Here's how the part is built. I have some questions about the finished solid (model axes, mm). A direction names the side the tool comes from. Round coordinates to 2 decimals unless told otherwise and drop trailing zeros. Write each loop counter-clockwise with the first axis right and the second up, starting at its lowest first coordinate (ties: lowest second). Pieces come first, ordered by that corner, then holes. Notation, with made-up numbers: (32.25, 54) -> (76.25, 54) arc R19 cw to (76.25, 74) -> close; hole circle Ø3 at (-36, 44). An arc over 180 degrees is marked (long way). Answer as CSV lines item,"result".
Solid Edge part; units mm, degrees
sketch "Sketch1" plane through (0, 0, 0) normal (0, 0, 1) x (1, 0, 0)
  line L0 (-7.7, -5.4) -> (7.7, -5.4)
  line L1 (7.7, -5.4) -> (7.7, -2.8)
  line L2 (7.7, -2.8) -> (9.7, -2.8)
  arc A0 (9.7, 2.8) -> (9.7, -2.8) centre (9.7, 0) cw
  line L3 (7.7, 2.8) -> (9.7, 2.8)
  line L4 (7.7, 5.4) -> (7.7, 2.8)
  line L5 (7.7, 5.4) -> (-7.7, 5.4)
  line L6 (-7.7, 5.4) -> (-7.7, 2.8)
  line L7 (-7.7, 2.8) -> (-9.7, 2.8)
  arc A1 (-9.7, 2.8) -> (-9.7, -2.8) centre (-9.7, 0) ccw
  line L8 (-7.7, -2.8) -> (-9.7, -2.8)
  line L9 (-7.7, -5.4) -> (-7.7, -2.8)
  dimension "D1" = 7.7
extrude "Protrusion1" add sketch "Sketch1" along normal blind 1.6
sketch "Sketch2" plane through (0, 0, 1.6) normal (0, 0, 1) x (1, 0, 0)
  circle A0 centre (9.65, 0) radius 1.45
  circle A1 centre (-9.65, 0) radius 1.45
extrude "Cutout1" cut sketch "Sketch2" against normal through all
sketch "Sketch3" plane through (0, 0, 1.6) normal (0, 0, 1) x (1, 0, 0)
  circle A0 centre (-6.25, -4.4) radius 0.5
  circle A1 centre (-3.75, -4.4) radius 0.5
  circle A2 centre (-1.25, -4.4) radius 0.5
  circle A3 centre (1.25, -4.4) radius 0.5
  circle A4 centre (3.75, -4.4) radius 0.5
  circle A5 centre (6.25, -4.4) radius 0.5
extrude "Cutout2" cut sketch "Sketch3" against normal through all
sketch "Sketch4" plane through (0, 0, 1.6) normal (0, 0, 1) x (1, 0, 0)
  line L0 (-2.5, 1.1) -> (2.5, 1.1)
  line L1 (2.5, 1.1) -> (2.5, 4.1)
  line L2 (2.5, 4.1) -> (-2.5, 4.1)
  line L3 (-2.5, 4.1) -> (-2.5, 1.1)
  dimension "D1" = 2.5
  dimension "D2" = 2.5
extrude "Extrusionsausprägung_2" add sketch "Sketch4" along normal blind 1.5
sketch "Sketch5" plane through (0, 0, 0) normal (0, 0, -1) x (-1, 0, 0)
  line L0 (-7.7, 5.4) -> (7.7, 5.4)
  line L1 (7.7, 5.4) -> (7.7, -2.9)
  line L2 (7.7, -2.9) -> (-7.7, -2.9)
  line L3 (-7.7, -2.9) -> (-7.7, 5.4)
extrude "Extrusionsausprägung_3" add sketch "Sketch5" along normal blind 1.5
Item 1: Suppose I cut it at B-B, the plane z = 0.65. State how many separate pieces and enclosed holes the cut face has, then the cut area to 3 significant figures.
Results found:
separate pieces,"1"
enclosed holes,"8"
area,"195 mm²"
Item 2: Suppose I cut it at A-A, the plane x = -6.25. List the corners of the cut face in (y, z) for me.
Results found:
outline,"(-5.4, 0) -> (-4.9, 0) -> (-4.9, 1.6) -> (-5.4, 1.6) -> close; (-3.9, 0) -> (-2.9, 0) -> (-2.9, -1.5) -> (5.4, -1.5) -> (5.4, 1.6) -> (-3.9, 1.6) -> close"
Item 3: Will these pins go through, and if not, where does the flat tip stop? pin 1 (4 mm diameter, centred on x = -9.65, y = 0, fed in from +Z); pin 2 (1.6 mm diameter, centred on y = 2, z = 2.5, fed in from +X); pin 3 (0.8 mm diameter, centred on x = -8.5, z = 0.5, fed in from -Y); pin 4 (1.7 mm diameter, centred on x = 9.65, y = 0, fed in from -Z).
Results found:
pin 1,"stops at z = 1.6"
pin 2,"stops at x = 2.5"
pin 3,"stops at y = -2.8"
pin 4,"passes through"
Item 4: For faces 4 (the flat face through (9, 2.8, 1)), 5 (the flat face through (-11, 1, 0)), 6 (the flat face through (2.5, 3, 2)), 7 (the flat face through (0, 1.1, 2)), 8 (the flat face through (0, -2.9, -1)), which set-ups out of +Z, -Z, +X, -X, +Y, -Y let a thin tool reach every point of the face, with its end or its side?
Results found:
face 4,"+Z, -Z, +X, +Y"
face 5,"-Z, -X, +Y, -Y"
face 6,"+Z, +X, +Y, -Y"
face 7,"+Z, +X, -X, -Y"
face 8,"-Z, +X, -X, -Y"
Item 5: Suppose I cut it at D-D, the plane x = -2. List the corners of the cut face in (y, z) for me.
Results found:
outline,"(-5.4, 0) -> (-2.9, 0) -> (-2.9, -1.5) -> (5.4, -1.5) -> (5.4, 1.6) -> (4.1, 1.6) -> (4.1, 3.1) -> (1.1, 3.1) -> (1.1, 1.6) -> (-5.4, 1.6) -> close"
Item 6: I need wall thicknesses on L1, parallel to Y at x = -1.25, z = 0.9; L2, parallel to Y at x = -9.65, z = 0.4; L3, parallel to Z at x = 2.5, y = 1. Which ranges of each line are inside material? Lowest first, please.
Results found:
L1,"y = -5.4 to -4.9, -3.9 to 5.4"
L2,"y = -2.8 to -1.45, 1.45 to 2.8"
L3,"z = -1.5 to 1.6"
Item 7: Suppose I cut it at C-C, the plane y = -4.4. List the corners of the cut face in (x, z) for me, then the cut area to 3 significant figures.
Results found:
outline,"(-7.7, 0) -> (-6.75, 0) -> (-6.75, 1.6) -> (-7.7, 1.6) -> close; (-5.75, 0) -> (-4.25, 0) -> (-4.25, 1.6) -> (-5.75, 1.6) -> close; (-3.25, 0) -> (-1.75, 0) -> (-1.75, 1.6) -> (-3.25, 1.6) -> close; (-0.75, 0) -> (0.75, 0) -> (0.75, 1.6) -> (-0.75, 1.6) -> close; (1.75, 0) -> (3.25, 0) -> (3.25, 1.6) -> (1.75, 1.6) -> close; (4.25, 0) -> (5.75, 0) -> (5.75, 1.6) -> (4.25, 1.6) -> close; (6.75, 0) -> (7.7, 0) -> (7.7, 1.6) -> (6.75, 1.6) -> close"
area,"15.0 mm²"
Item 8: If we mould it in two halves opening along X, with no side actions, what happens to faces 1 (the flat face through (-2.5, 3, 2)), 2 (the cylindrical face through (12.5, 0.1, 0.8)), 3 (the cylindrical face through (-8.311, -0.555, 0.811))? For each: pulls with the +X half, pulls with the -X half, needs draft (parallel to the pull), parting line crosses it, or undercut.
Results found:
face 1,"pulls with the -X half"
face 2,"pulls with the +X half"
face 3,"undercut"
